The listing builds one solid part. Answer for the finished solid, in the listing's coordinates (mm). Coordinates: 2 decimals unless noted, no trailing zeros. Loops run counter-clockwise (first coordinate to the right, second up) from the corner with the lowest first, then second, coordinate; pieces in that order, holes last. Notation, with made-up numbers: M 37.5,-33.75 L 90.5,-33.75 A19 cw 90.5,-18.75 Z; hole C -34.5,-25 d6. An arc over 180 degrees is marked long. Answer as a JSON object with one key per item and string values. Group by question number.
1. Determine the mould class of faces 1 (the face through (34.73, -12.85, 1.57)), 2 (the face through (0, -26, 2)), 3 (the face through (51, -38, 2)), 4 (the face through (12, -16, 2)) for opening direction Y: released by +Y, released by -Y, zero draft, split by the parting line, or undercut.
2. Given pin 1 (6 mm diameter, centred on x = 63.5, y = -12.7, fed in from +Z); pin 2 (1 mm diameter, centred on y = -41.5, z = 1, fed in from +X); pin 3 (1 mm diameter, centred on x = 47.5, z = 0.5, fed in from -Y), each flat-ended and moving along its own axis, determine where each tip first touches the part or whether it passes through.
3. A cutting plane is placed at B-B on y = -38.1. Give the vertices of the cut face in (x, z) (3 decimals), and give its area (3 significant figures).
4. A cutting plane is placed at D-D on z = 1. Give the vertices of the cut face in (x, y), and give its area (3 significant figures).
5. A cutting plane is placed at A-A on x = 63.5. Give the vertices of the cut face in (y, z) (3 decimals).
6. A cutting plane is placed at C-C on x = 12.7. Give the vertices of the cut face in (y, z) (3 decimals), and give its area (3 significant figures).
7. Straight lines are drawn through the part: L1, parallel to Y at x = 12.7, z = 1.45; L2, parallel to X at y = -10, z = 1.2; L3, parallel to X at y = -35, z = 1.25. For each, find the intervals that lie inside material, in ascending order.
Autodesk Inventor part; units mm, degrees
ref_plane "YZ Plane" through (0, 0, 0) normal (1, 0, 0) x (0, 1, 0)
ref_plane "XZ Plane" through (0, 0, 0) normal (0, 1, 0) x (-1, 0, 0)
ref_plane "XY Plane" through (0, 0, 0) normal (0, 0, 1) x (1, 0, 0)
sketch "Sketch1" plane through (0, 0, 0) normal (0, 0, 1) x (1, 0, 0)
  line L0 (0, 0) -> (76.2, 0)
  line L1 (76.2, 0) -> (76.2, -25.4)
  line L2 (76.2, -25.4) -> (25.4, -50.8)
  line L3 (25.4, -50.8) -> (0, -50.8)
  line L4 (0, -50.8) -> (0, 0)
  circle A0 centre (63.5, -12.7) radius 3.3734
  circle A1 centre (38.1, -12.7) radius 3.3734
  circle A2 centre (12.7, -12.7) radius 3.3734
  circle A3 centre (12.7, -38.1) radius 3.3734
  dimension "d0" = 25.4
  dimension "d1" = 25.4
  dimension "d2" = 76.2
  dimension "d3" = 50.8
  dimension "d4" = 6.7469
  dimension "d5" = 12.7
  dimension "d6" = 12.7
  dimension "d7" = 12.7
  dimension "d8" = 12.7
  dimension "d9" = 12.7
  dimension "d10" = 38.1
  dimension "d11" = 12.7
  dimension "d12" = 12.7
extrude "Extrusion1" add sketch "Sketch1" along normal blind 3.175
properties part number "bottom gusset"
From the geometry:
{
 "1": {"face 1": "undercut", "face 2": "zero draft", "face 3": "released by -Y", "face 4": "undercut"},
 "2": {"pin 1": "passes through", "pin 2": "stops at x = 45", "pin 3": "stops at y = -40"},
 "3": {"outline": "M 0,0 L 9.327,0 L 9.327,3.175 L 0,3.175 Z; M 16.073,0 L 50.8,0 L 50.8,3.175 L 16.073,3.175 Z", "area": "140 mm²"},
 "4": {"outline": "M 0,-50.8 L 25.4,-50.8 L 76.2,-25.4 L 76.2,0 L 0,0 Z; hole C 12.7,-38.1 d6.75; hole C 12.7,-12.7 d6.75; hole C 38.1,-12.7 d6.75; hole C 63.5,-12.7 d6.75", "area": "3,080 mm²"},
 "5": {"outline": "M -31.75,0 L -16.073,0 L -16.073,3.175 L -31.75,3.175 Z; M -9.327,0 L 0,0 L 0,3.175 L -9.327,3.175 Z"},
 "6": {"outline": "M -50.8,0 L -41.473,0 L -41.473,3.175 L -50.8,3.175 Z; M -34.727,0 L -16.073,0 L -16.073,3.175 L -34.727,3.175 Z; M -9.327,0 L 0,0 L 0,3.175 L -9.327,3.175 Z", "area": "118 mm²"},
 "7": {"L1": "y = -50.8 to -41.47, -34.73 to -16.07, -9.33 to 0", "L2": "x = 0 to 10.68, 14.72 to 36.08, 40.12 to 61.48, 65.52 to 76.2", "L3": "x = 0 to 11.37, 14.03 to 57"}
}
